Check sheet for the drawn part. Datum: minimum x, y, z corner. Units: mm. A direction names the side the tool comes from. Round coordinates to 2 decimals unless told otherwise and drop trailing zeros. Order: outer loops, then holes, each group sorted by start corner. A loop starts at its lowest first (then second) coordinate and runs counter-clockwise, first axis right, second up. Notation, with made-up numbers: (-16, -7.5) -> (18, -7.5) arc R20 ccw to (18, 21.5) -> close; hole circle Ø4 at (86.25, -2.75). An arc over 180 degrees is marked (long way). Use CSV: the item, a comma, the result in double quotes.
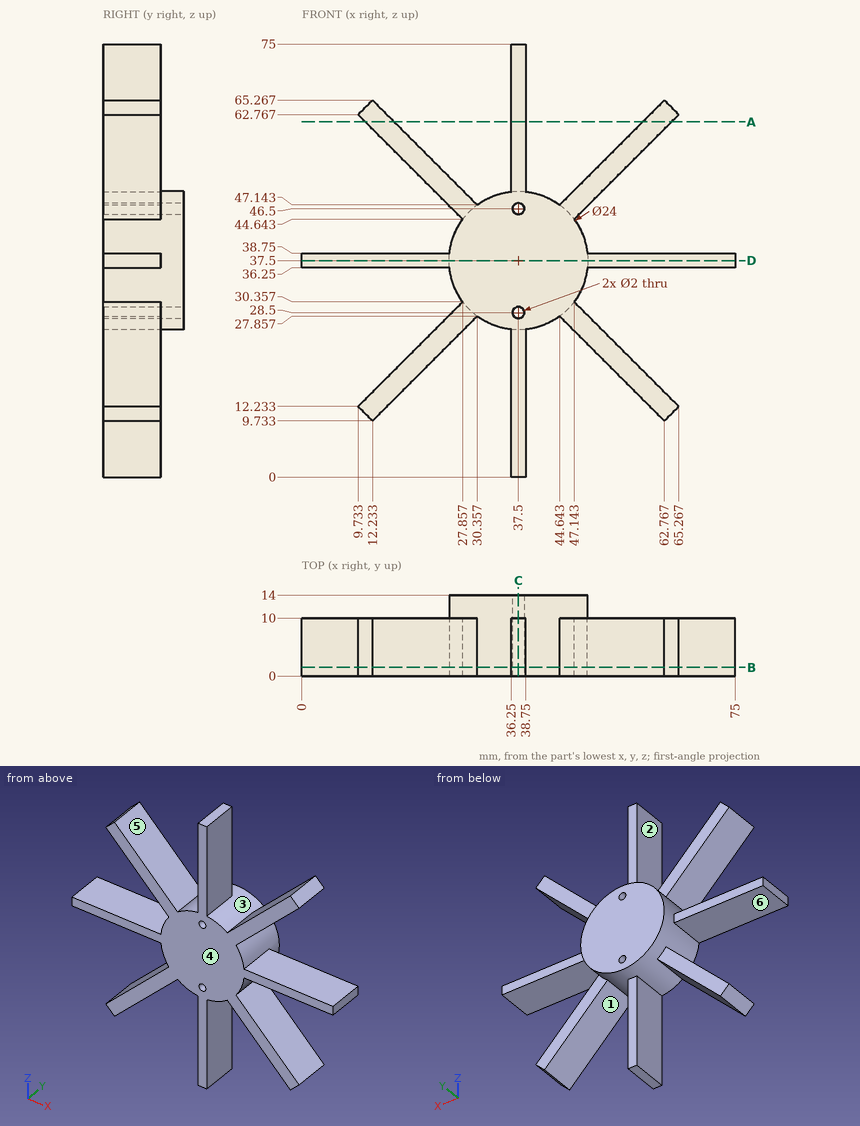
Q1. Go/stop test with flat-tipped pins: pin 1 (2 mm diameter, centred on x = 19.5, y = 7.5, fed in from +Z); pin 2 (3 mm diameter, centred on x = 11.5, z = 38, fed in from +Y); pin 3 (3 mm diameter, centred on x = 56, y = 2.5, fed in from +Z). Record where each tip stops, or that it passes through.
Result sheet:
pin 1,"stops at z = 59"
pin 2,"stops at y = 10"
pin 3,"stops at z = 60"
Q2. Mould release check, pull along Z, two halves, no side actions. Record for the marked faces 4, 5 and 6: pulls with the +Z half, pulls with the -Z half, needs draft (parallel to the pull), parting line crosses it, or undercut.
Result sheet:
face 4,"needs draft"
face 5,"pulls with the +Z half"
face 6,"undercut"
Q3. Scan lines: L1, parallel to Z at x = 37.5, y = 4.25; L2, parallel to Z at x = 37.5, y = 11; L3, parallel to X at y = 5, z = 48 (1 decimal). Record each from-to range of solid material in increasing order.
Result sheet:
L1,"z = 0 to 27.5, 29.5 to 45.5, 47.5 to 75"
L2,"z = 25.5 to 27.5, 29.5 to 45.5, 47.5 to 49.5"
L3,"x = 24.5 to 29.5, 31.7 to 43.3, 45.5 to 50.5"
Q4. Sectioned sample at D-D, the plane z = 37.5. Enter the section's corners in (x, y), then the cut area to 3 significant figures.
Result sheet:
outline,"(0, 0) -> (75, 0) -> (75, 10) -> (49.5, 10) -> (49.5, 14) -> (25.5, 14) -> (25.5, 10) -> (0, 10) -> close"
area,"846 mm^2"
Q5. Sectioned sample at C-C, the plane x = 37.5. Enter the section's corners in (y, z).
Result sheet:
outline,"(0, 0) -> (10, 0) -> (10, 25.5) -> (14, 25.5) -> (14, 27.5) -> (0, 27.5) -> close; (0, 29.5) -> (14, 29.5) -> (14, 45.5) -> (0, 45.5) -> close; (0, 47.5) -> (14, 47.5) -> (14, 49.5) -> (10, 49.5) -> (10, 75) -> (0, 75) -> close"
Q6. Access from +Z, -Z, +X, -X, +Y, -Y to the whole of each face (thin tool, end or side, straight path). Record for the marked faces 1, 2 and 3.
Result sheet:
face 1,"-Z, +Y, -Y"
face 2,"+Z, +Y, -Y"
face 3,"+Y"
Q7. Sectioned sample at A-A, the plane z = 61.5. Enter the section's corners in (x, y), then the cut area to 3 significant figures.
Result sheet:
outline,"(11, 0) -> (16, 0) -> (16, 10) -> (11, 10) -> close; (36.25, 0) -> (38.75, 0) -> (38.75, 10) -> (36.25, 10) -> close; (59, 0) -> (64, 0) -> (64, 10) -> (59, 10) -> close"
area,"125 mm^2"
Q8. Sectioned sample at B-B, the plane y = 1.5. State how many separate pieces and enclosed holes the cut face has, then the cut area to 3 significant figures.
Result sheet:
separate pieces,"1"
enclosed holes,"2"
area,"1,060 mm^2"
